Geometry: final body of the model. Coordinates: model frame, mm. Face numbers are marked on the shaded views. A direction names the side the tool comes from. Coordinates: 2 decimals unless noted, no trailing zeros. Order: outer loops, then holes, each group sorted by start corner. A loop starts at its lowest first (then second) coordinate and runs counter-clockwise, first axis right, second up. Notation, with made-up numbers: (-39.75, 16.25) - (-17.75, 16.25) arc R18 ccw to (-17.75, 37.25) - close; hole circle Ø11 at (9, 79). An arc over 180 degrees is marked (long way). Use a Markdown table: item, result. Add a question column.
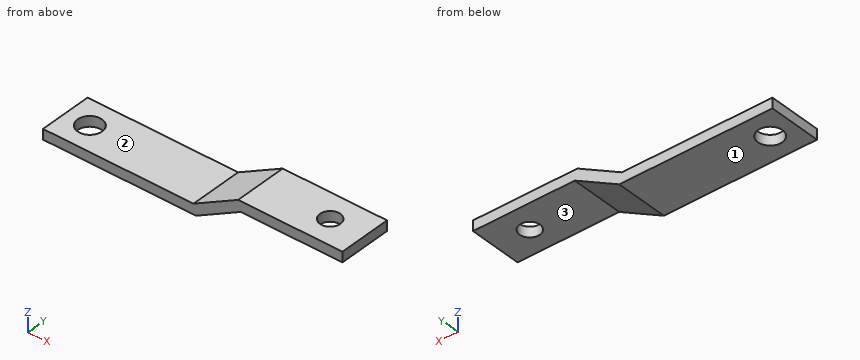
```python
from build123d import *

# Parameters (mm, degrees)
EXTRUDE_THIN1_DEPTH = 13.208
CUT_EXTRUDE1_REACH  = 10.669
SKETCH3_R           = 3.048
CUT_EXTRUDE2_REACH  = 10.669
SKETCH4_R           = 2.54


with BuildPart() as part:
    # Sketch1 → Extrude-Thin1 (new body)
    with BuildSketch(Plane(origin=(0, 0, 0), x_dir=(1, 0, 0), z_dir=(0, 1, 0))):
        Polygon((0, 0), (38.139058105, 0), (49.245270394, -6.128868698), (74.567434413, -6.128868698), (74.567434413, -8.668868698), (48.590941352, -8.668868698), (37.484729063, -2.54), (0, -2.54), align=None)
    extrude(amount=EXTRUDE_THIN1_DEPTH)

    # Sketch3 → Cut-Extrude1 (cut, up to next)
    with BuildSketch(Plane(origin=(0, 0, 0), x_dir=(-1, 0, 0), z_dir=(0, 0, -1)), mode=Mode.PRIVATE) as cut_extrude1_sk1:
        with Locations((-6.110625798, 6.604)):
            Circle(SKETCH3_R)
    cut_extrude1_tool1 = extrude(cut_extrude1_sk1.sketch, amount=-CUT_EXTRUDE1_REACH, mode=Mode.PRIVATE) & part.part
    add(cut_extrude1_tool1.solids().sort_by_distance((6.110626, 6.604, 0))[0], mode=Mode.SUBTRACT)

    # Sketch4 → Cut-Extrude2 (cut, up to next)
    with BuildSketch(Plane.XY.offset(8.668868698), mode=Mode.PRIVATE) as cut_extrude2_sk1:
        with Locations((65.966386127, 6.604)):
            Circle(SKETCH4_R)
    cut_extrude2_tool1 = extrude(cut_extrude2_sk1.sketch, amount=-CUT_EXTRUDE2_REACH, mode=Mode.PRIVATE) & part.part
    add(cut_extrude2_tool1.solids().sort_by_distance((65.966386, 6.604, 8.668869))[0], mode=Mode.SUBTRACT)


solid = part.part
```
1) Ray query, line 1 along Z through (x, y) = (52, 9); line 2 along Z through (x, y) = (13, 8.5); line 3 along Y through (x, z) = (5.5, 2.5). Return the intervals inside material, ascending.
2) Pin query (flat end, axial travel): pin 1 (6.5 mm diameter, centred on x = 65.97, y = 6.6, fed in from +Z); pin 2 (4 mm diameter, centred on x = 11.5, y = 7.5, fed in from +Z); pin 3 (2 mm diameter, centred on x = 24, z = 5, fed in from -Y); pin 4 (4 mm diameter, centred on x = 63.5, y = 9, fed in from -Z). Return the tip coordinate at first contact, or that it passes through.
3) Set-up query: the marked faces 1, 2 and 3. Return all of +Z, -Z, +X, -X, +Y, -Y with unobstructed straight access to the full face (end or side cutting, diameter ignored); none if empty.
4) Section D-D (z = 8). Return loops of the section in (x, y), then the cut area to 3 significant figures.
5) Section C-C (y = 11). Return loops of the section in (x, z).
6) Section B-B (y = 5.75). Return loops of the section in (x, z).
7) Section A-A (x = 7). Return loops of the section in (y, z), then the cut area to 3 significant figures.
Values follow:
| question | item | result |
|---|---|---|
| 1 | line 1 | z = 6.13 to 8.67 |
| 1 | line 2 | z = 0 to 2.54 |
| 1 | line 3 | y = 0 to 3.62, 9.59 to 13.21 |
| 2 | pin 1 | stops at z = 8.67 |
| 2 | pin 2 | stops at z = 2.54 |
| 2 | pin 3 | passes through |
| 2 | pin 4 | stops at z = 6.13 |
| 3 | face 1 | -Z, +X, -X, +Y, -Y |
| 3 | face 2 | +Z, -X, +Y, -Y |
| 3 | face 3 | -Z, +X, +Y, -Y |
| 4 | outline | (47.38, 0) - (74.57, 0) - (74.57, 13.21) - (47.38, 13.21) - close; hole circle Ø5.08 at (65.97, 6.6) |
| 4 | area | 339 mm² |
| 5 | outline | (0, 0) - (38.14, 0) - (49.25, 6.13) - (74.57, 6.13) - (74.57, 8.67) - (48.59, 8.67) - (37.48, 2.54) - (0, 2.54) - close |
| 6 | outline | (0, 0) - (3.18, 0) - (3.18, 2.54) - (0, 2.54) - close; (9.04, 0) - (38.14, 0) - (49.25, 6.13) - (63.57, 6.13) - (63.57, 8.67) - (48.59, 8.67) - (37.48, 2.54) - (9.04, 2.54) - close; (68.36, 6.13) - (74.57, 6.13) - (74.57, 8.67) - (68.36, 8.67) - close |
| 7 | outline | (0, 0) - (3.69, 0) - (3.69, 2.54) - (0, 2.54) - close; (9.52, 0) - (13.21, 0) - (13.21, 2.54) - (9.52, 2.54) - close |
| 7 | area | 18.7 mm² |
